Here's the drawing with two shaded views (mm, measured from the low corner). I have some questions. A direction names the side the tool comes from. Give positions to 0.01 mm unless a question says otherwise; leave off trailing zeros. Order: outer loops, then holes, each group sorted by start corner. A loop starts at its lowest first (then second) coordinate and runs counter-clockwise, first axis right, second up. Notation, with made-up numbers: (9, -28.75) - (39, -28.75) arc R14 ccw to (39, -24.75) - close; hole circle Ø8 at (81, -29). An arc over 180 degrees is marked (long way). Use one line per item in the form item = value. Start each with the question number.
1) We'd pull the mould along Z, two halves only. Please class the marked faces 3, 4 and 5: released by +Z, released by -Z, zero draft, split by the parting line, or undercut.
2) Suppose I cut it at A-A, the plane y = 70. Write out the boundary of the cut face in (x, z), and give its area (3 significant figures).
3) Which directions (+Z, -Z, +X, -X, +Y, -Y) give clear straight access to the entire face, cutting with the end or side of a thin tool? Please do the marked faces 1 and 2.
4) Suppose I cut it at C-C, the plane z = 550.5. Write out the boundary of the cut face in (x, y), and give its area (3 significant figures).
5) Please list where these lines run through material, in increasing order: probe 1 along Y at (x, z) = (561, 741); probe 2 along Z at (x, y) = (54.5, 546).
6) Suppose I cut it at D-D, the plane y = 549.5. Write out the boundary of the cut face in (x, z).
7) Suppose I cut it at B-B, the plane x = 348.5. Write out the boundary of the cut face in (y, z).
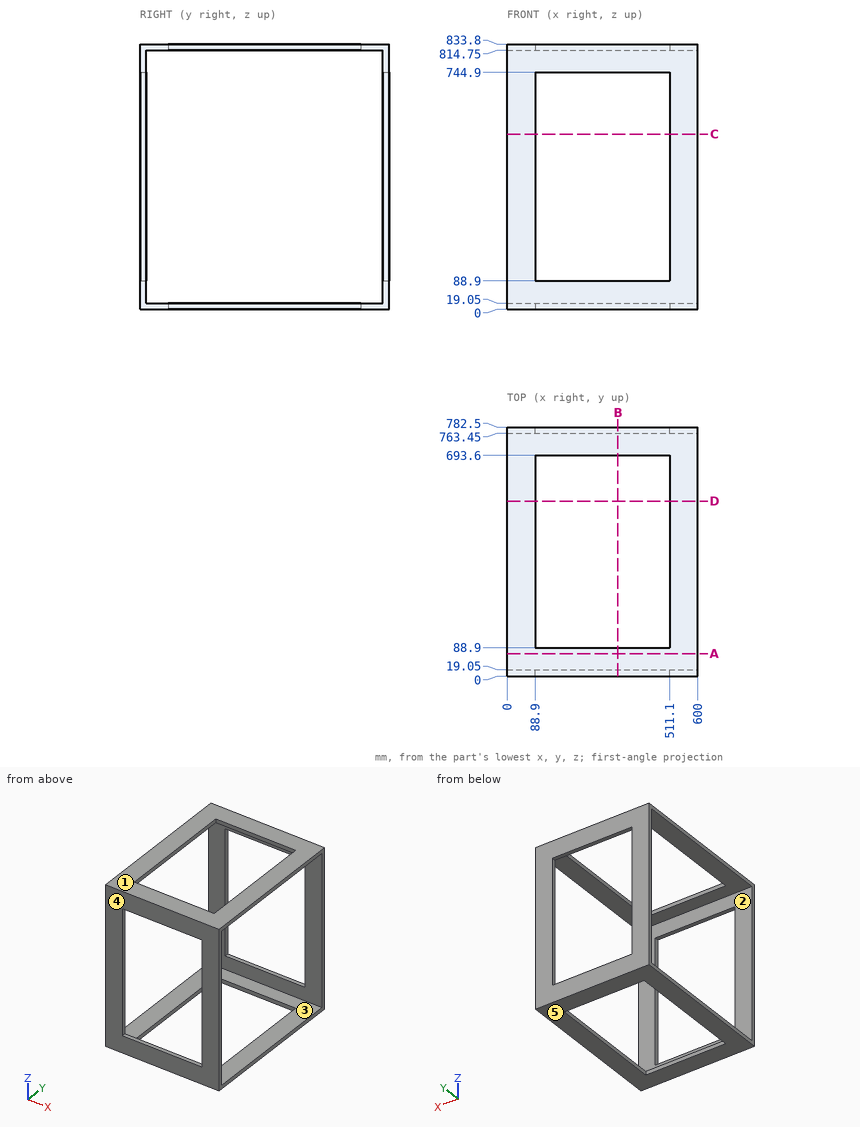
Result sheet:
q1.face_3 = undercut
q1.face_4 = zero draft
q1.face_5 = released by -Z
q2.outline = (0, 0) - (600, 0) - (600, 19.05) - (0, 19.05) - close; (0, 814.75) - (600, 814.75) - (600, 833.8) - (0, 833.8) - close
q2.area = 22,900 mm²
q3.face_1 = +Z, +X, -X, +Y, -Y
q3.face_2 = +X, -X
q4.outline = (0, 0) - (88.9, 0) - (88.9, 19.05) - (0, 19.05) - close; (0, 763.45) - (88.9, 763.45) - (88.9, 782.5) - (0, 782.5) - close; (511.1, 0) - (600, 0) - (600, 19.05) - (511.1, 19.05) - close; (511.1, 763.45) - (600, 763.45) - (600, 782.5) - (511.1, 782.5) - close
q4.area = 6,770 mm²
q5.probe_1 = 0 to 19.05, 763.45 to 782.5
q5.probe_2 = 0 to 19.05, 814.75 to 833.8
q6.outline = (0, 0) - (88.9, 0) - (88.9, 19.05) - (0, 19.05) - close; (0, 814.75) - (88.9, 814.75) - (88.9, 833.8) - (0, 833.8) - close; (511.1, 0) - (600, 0) - (600, 19.05) - (511.1, 19.05) - close; (511.1, 814.75) - (600, 814.75) - (600, 833.8) - (511.1, 833.8) - close
q7.outline = (0, 0) - (88.9, 0) - (88.9, 19.05) - (19.05, 19.05) - (19.05, 88.9) - (0, 88.9) - close; (0, 744.9) - (19.05, 744.9) - (19.05, 814.75) - (88.9, 814.75) - (88.9, 833.8) - (0, 833.8) - close; (693.6, 0) - (782.5, 0) - (782.5, 88.9) - (763.45, 88.9) - (763.45, 19.05) - (693.6, 19.05) - close; (693.6, 814.75) - (763.45, 814.75) - (763.45, 744.9) - (782.5, 744.9) - (782.5, 833.8) - (693.6, 833.8) - close
